Verification items for the finished model (mm, model axes). A direction names the side the tool comes from. Give positions to 0.01 mm unless a question says otherwise; leave off trailing zeros. Order: outer loops, then holes, each group sorted by start corner. A loop starts at its lowest first (then second) coordinate and runs counter-clockwise, first axis right, second up.
(1) Sectioned sample at A-A on z = 3. Record the cut outline in (x, y).
(2) Gauge pin test, flat ends, axial feed: pin 1 (5 mm diameter, centred on x = 1.5, z = 5, fed in from +Y); pin 2 (2 mm diameter, centred on x = -1, z = 2, fed in from -Y); pin 3 (1.5 mm diameter, centred on x = 4, y = -6, fed in from -Z). Record the tip position at first contact, or that the pin passes through.
(3) Sectioned sample at B-B on z = 13.5. Record the cut outline in (x, y), plus the area to 3 significant figures.
(4) Scan lines: L1, parallel to X at y = -5, z = 12; L2, parallel to X at y = -2.25, z = 5.75; L3, parallel to Z at x = -4.75, y = -0.5. Record each from-to range of solid material in increasing order.
(5) Access from +Z, -Z, +X, -X, +Y, -Y to the whole of each face (thin tool, end or side, straight path). Record for faces 1 (the face through (0.11, -5.05, 1.86)), 2 (the face through (0, 0, 3)).
```python
from build123d import *

# Parameters (mm, degrees)
F1_ANGLE = 180
F2_R     = 4


with BuildPart() as f1:
    # F0 (on Front) → F1 (revolve)
    with BuildSketch(Plane.XZ):
        with BuildLine():
            ThreePointArc((0, 16.6), (4.6669047558, 14.6669047558), (6.6, 10))
            ThreePointArc((6.6, 10), (6.2004032127, 7.7383634244), (5.05, 5.750588276))
            Line((5.05, 5.750588276), (5.05, 5.0806504495))
            ThreePointArc((5.05, 5.0806504495), (6.5308881479, 7.3448163905), (7.05, 10))
            ThreePointArc((7.05, 10), (4.9851028074, 14.9851028074), (0, 17.05))
            Line((0, 17.05), (0, 16.6))
        make_face()
        with BuildLine():
            Line((5.05, 5.0806504495), (5.05, 5.750588276))
            ThreePointArc((5.05, 5.750588276), (2.7851285986, 4.016434283), (0, 3.4))
            Line((0, 3.4), (0, 2.95))
            ThreePointArc((0, 2.95), (2.740536961, 3.5044663679), (5.05, 5.0806504495))
        make_face()
        with BuildLine():
            Line((5.05, 0), (5.05, 5.0806504495))
            ThreePointArc((5.05, 5.0806504495), (2.740536961, 3.5044663679), (0, 2.95))
            Line((0, 2.95), (0, 0))
            Line((0, 0), (5.05, 0))
        make_face()
    revolve(axis=Axis((0, 0, 10), (0, 0, -1)), revolution_arc=F1_ANGLE)

    # F2
    f2_edges = [f1.edges().sort_by_distance(p)[0] for p in [
        (0, -5.05, 5.08065),
    ]]
    fillet(f2_edges, radius=F2_R)


solid = f1.part
```
Ans:
1. outline: (-5.05, 0) arc R5.05 ccw to (5.05, 0) - close
2. pin 1: stops at y = 0
2. pin 2: stops at y = -5.05
2. pin 3: stops at z = 7.18
3. outline: (-6.12, 0) arc R6.12 ccw to (6.12, 0) - (5.6, 0) arc R5.6 cw to (-5.6, 0) - close
3. area: 9.65 mm2
4. L1: x = -4.55 to -3.82, 3.82 to 4.55
4. L2: x = -5.17 to -4.52, 4.52 to 5.17
4. L3: z = 0 to 5.45, 14.55 to 15.19
5. face 1: -Z, -Y
5. face 2: +Z, -Z, +X, -X, +Y
